```python
from build123d import *

# Parameters (mm, degrees)
F0_R     = 7.5
F1_DEPTH = 4
F2_R     = 5
F3_DEPTH = 100
F4_W     = 2
F4_H     = 4
F5_DEPTH = 20


with BuildPart() as f1:
    # F0 (on Top) → F1 (new body)
    with BuildSketch(Plane.XY):
        Circle(F0_R)
    extrude(amount=F1_DEPTH)

    # F2 (on Top) → F3 (join)
    with BuildSketch(Plane.XY):
        Circle(F2_R)
    extrude(amount=F3_DEPTH)

    # F4 (on face) → F5 (join)
    with BuildSketch(Plane.XY.offset(100)):
        Rectangle(F4_W, F4_H)
    extrude(amount=F5_DEPTH)


solid = f1.part
```
Check sheet for the modelled part. Datum: model origin and axes. Units: mm. A direction names the side the tool comes from. Round coordinates to 2 decimals unless told otherwise and drop trailing zeros. Order: outer loops, then holes, each group sorted by start corner. A loop starts at its lowest first (then second) coordinate and runs counter-clockwise, first axis right, second up.
1) Go/stop test with flat-tipped pins: pin 1 Ø4 at (x, z) = (4.5, 51.5) entering from +Y; pin 2 Ø0.6 at (x, z) = (-0.5, 113) entering from +Y; pin 3 Ø4.5 at (y, z) = (-0.5, 111) entering from +X. Record where each tip stops, or that it passes through.
2) Section check D-D (z = 69.5). Record the boundary of the cut face in (x, y), and give its area (3 significant figures).
3) Section check C-C (z = 106.5). Record the boundary of the cut face in (x, y).
4) Scan lines: line 1 (Z direction, x = -1.25, y = 0.75); line 2 (Z direction, x = -2.5, y = 6.25); line 3 (Y direction, x = -0.5, z = 36). Record each from-to range of solid material in increasing order.
5) Section check A-A (x = 0). Record the boundary of the cut face in (y, z).
6) Tool access check on faces 1 (the flat face through (-1, 0, 110)), 2 (the cylindrical face through (-1.08, -4.88, 51.33)), 3 (the flat face through (1, 0, 110)), 4 (the flat face through (0, 2, 110)), 5 (the flat face through (0, -2, 110)). Record the directions out of +Z, -Z, +X, -X, +Y, -Y that give a thin tool (end or side, any length) a straight path to the whole face; none if there is none.
7) Section check B-B (y = 0). Record the boundary of the cut face in (x, z).
Result:
1. pin 1: stops at y = 4.33
1. pin 2: stops at y = 2
1. pin 3: stops at x = 1
2. outline: circle Ø10 at (0, 0)
2. area: 78.5 mm2
3. outline: (-1, -2) - (1, -2) - (1, 2) - (-1, 2) - close
4. line 1: z = 0 to 100
4. line 2: z = 0 to 4
4. line 3: y = -4.97 to 4.97
5. outline: (-7.5, 0) - (7.5, 0) - (7.5, 4) - (5, 4) - (5, 100) - (2, 100) - (2, 120) - (-2, 120) - (-2, 100) - (-5, 100) - (-5, 4) - (-7.5, 4) - close
6. face 1: +Z, -X, +Y, -Y
6. face 2: +Z
6. face 3: +Z, +X, +Y, -Y
6. face 4: +Z, +X, -X, +Y
6. face 5: +Z, +X, -X, -Y
7. outline: (-7.5, 0) - (7.5, 0) - (7.5, 4) - (5, 4) - (5, 100) - (1, 100) - (1, 120) - (-1, 120) - (-1, 100) - (-5, 100) - (-5, 4) - (-7.5, 4) - close
